Geometry: final body of the model. Coordinates: model frame, mm. A direction names the side the tool comes from. Coordinates: 2 decimals unless noted, no trailing zeros. Order: outer loops, then holes, each group sorted by start corner. A loop starts at its lowest first (then second) coordinate and runs counter-clockwise, first axis right, second up. Notation, with made-up numbers: (-5.75, 72) -> (34.25, 72) arc R34 cw to (34.25, 102) -> close; hole circle Ø4 at (19.5, 16). An arc over 180 degrees is marked (long way). Use one line per item in the form item = value.
```python
from build123d import *

# Parameters (mm, degrees)
F0_W     = 83.6
F0_H     = 3
F0_H_2   = 8.4
F0_H_3   = 12
F1_DEPTH = 2
F2_DEPTH = 6
F3_R     = 2
F4_R     = 5
F5_R     = 1


with BuildPart() as f1:
    # F0 (on Top) → F1 (new body)
    with BuildSketch(Plane.XY):
        with Locations((41.8, 9.9)):
            Rectangle(F0_W, F0_H)
        with Locations((41.8, -1.5)):
            Rectangle(F0_W, F0_H)
        with Locations((41.8, 4.2)):
            Rectangle(F0_W, F0_H_2)
        with Locations((41.8, 17.4)):
            Rectangle(F0_W, F0_H_3)
        with Locations((41.8, -9)):
            Rectangle(F0_W, F0_H_3)
    extrude(amount=-F1_DEPTH)

    # F0 (on Top) → F2 (join)
    with BuildSketch(Plane.XY):
        with Locations((41.8, 9.9)):
            Rectangle(F0_W, F0_H)
        with Locations((41.8, -1.5)):
            Rectangle(F0_W, F0_H)
    extrude(amount=F2_DEPTH)

    # F3
    f3_edges = [f1.edges().sort_by_distance(p)[0] for p in [
        (0, 9.9, 6),
        (0, -1.5, 6),
        (83.6, 9.9, 6),
        (83.6, -1.5, 6),
    ]]
    fillet(f3_edges, radius=F3_R)

    # F4
    f4_edges = [f1.edges().sort_by_distance(p)[0] for p in [
        (83.6, -15, -1),
        (83.6, 23.4, -1),
        (0, 23.4, -1),
        (0, -15, -1),
    ]]
    fillet(f4_edges, radius=F4_R)

    # F5
    f5_edges = [f1.edges().sort_by_distance(p)[0] for p in [
        (41.8, 23.4, -2),
    ]]
    fillet(f5_edges, radius=F5_R)


solid = f1.part
```
1) Access query for faces 4 (the flat face through (41, 8.4, 3)), 5 (the flat face through (41, -3, 3)), 6 (the flat face through (41, 17, 0)). Directions: +Z, -Z, +X, -X, +Y, -Y. A direction counts if a zero-diameter tool reaches every point of the face in a straight line with its end or side. Return the directions, or none.
Results found:
face_4 = +Z, +X, -X
face_5 = +Z, +X, -X, -Y
face_6 = +Z, +X, -X, +Y
2) Section D-D, the plane z = 5.25. Output: boundary loops of the cut face in (x, y).
Results found:
outline = (0.44, -3) -> (83.16, -3) -> (83.16, 0) -> (0.44, 0) -> close; (0.44, 8.4) -> (83.16, 8.4) -> (83.16, 11.4) -> (0.44, 11.4) -> close
3) Section B-B, the plane x = 27.5. Output: boundary loops of the cut face in (y, z), and give its area (3 significant figures).
Results found:
outline = (-15, -1) arc R1 ccw to (-14, -2) -> (22.4, -2) arc R1 ccw to (23.4, -1) -> (23.4, 0) -> (11.4, 0) -> (11.4, 6) -> (8.4, 6) -> (8.4, 0) -> (0, 0) -> (0, 6) -> (-3, 6) -> (-3, 0) -> (-15, 0) -> close
area = 112 mm2
4) Contact query for flat-ended pins moving along their axis: P1, Ø1.8, axis at x = 49, z = 3, coming from the +Y side; P2, Ø3.5, axis at x = 39, y = 20.5, coming from the +Z side. Output: stop coordinate, or through.
Results found:
P1 = 11.4
P2 = 0
5) Section A-A, the plane z = 1.25. Output: boundary loops of the cut face in (x, y), and give its area (3 significant figures).
Results found:
outline = (0, -3) -> (83.6, -3) -> (83.6, 0) -> (0, 0) -> close; (0, 8.4) -> (83.6, 8.4) -> (83.6, 11.4) -> (0, 11.4) -> close
area = 502 mm2
6) Pull-direction query (Y, two-part tool) for faces 1 (the flat face through (41, 4, 0)), 2 (the flat face through (41, -9, 0)), 3 (the cylindrical face through (82.1, 21.97, -0.51)); classes: released by +Y, released by -Y, zero draft, split by the parting line, or undercut.
Results found:
face_1 = undercut
face_2 = zero draft
face_3 = released by +Y
7) Section C-C, the plane y = -6.5. Output: boundary loops of the cut face in (x, z), and give its area (3 significant figures).
Results found:
outline = (0, -1) arc R1 ccw to (1, -2) -> (82.6, -2) arc R1 ccw to (83.6, -1) -> (83.6, 0) -> (0, 0) -> close
area = 167 mm2
8) Material intervals for probe 1 along Y at (x, z) = (11, 3.25); probe 2 along Z at (x, y) = (19.5, 15.5); probe 3 along X at (y, z) = (9.5, 5), sorted ascending. Write a range as from..to.
Results found:
probe_1 = -3..0, 8.4..11.4
probe_2 = -2..0
probe_3 = 0.27..83.33
